Could you check a few things on this model? Use its own coordinates, in mm. Round coordinates to 2 decimals unless told otherwise and drop trailing zeros. Loops run counter-clockwise (first coordinate to the right, second up) from the corner with the lowest first, then second, coordinate; pieces in that order, holes last. Notation, with made-up numbers: M -22,-2.75 L -10,-2.75 A30 cw -10,23.25 Z; hole C 5.25,-18 d4. An arc over 180 degrees is marked long. One line per item, written item: value. Start each with the question number.
Q1. Imagine slicing it at A-A (x = 42). Please give me the cut outline in (y, z).
Q2. I'm going to push flat-ended pins straight in: pin 1 Ø1.6 at (y, z) = (-8.5, 2) entering from +X; pin 2 Ø1.6 at (y, z) = (12.5, 2) entering from -X; pin 3 Ø1.6 at (x, z) = (-1, 1.5) entering from -Y. Where does each tip first touch, or does it pass through?
Q3. Imagine slicing it at B-B (z = 0.7). Give the number of separate pieces and of enclosed holes in the cut face, then the cut area to 3 significant figures.
Q4. Please list where these lines run through material, in increasing order: line 1 along X through (y, z) = (12.25, 0.75); line 2 along X through (y, z) = (0.75, 1.25); line 3 along X through (y, z) = (2.75, 0.8).
from build123d import *

# Parameters (mm, degrees)
SKETCH1_R           = 1.4
BOSS_EXTRUDE1_DEPTH = 3.15
SKETCH2_R           = 1.4
CUT_EXTRUDE1_DEPTH  = 10


with BuildPart() as part:
    # Sketch1 → Boss-Extrude1 (new body)
    with BuildSketch(Plane.XY):
        Polygon((-60.67170061, 10.980201327), (-60.67170061, -7.339798673), (-35.52170061, -7.339798673), (-35.52170061, -7.389798673), (-35.52170061, -10.539798673), (-15.62170061, -10.539798673), (-15.62170061, -7.339798673), (4.47829939, -7.339798673), (4.47829939, -10.539798673), (24.37829939, -10.539798673), (24.37829939, -7.339798673), (44.47829939, -7.339798673), (44.47829939, -10.539798673), (64.37829939, -10.539798673), (64.37829939, -7.339798673), (84.47829939, -7.339798673), (84.47829939, -10.539798673), (104.37829939, -10.539798673), (104.37829939, -7.339798673), (124.47829939, -7.339798673), (124.47829939, -10.539798673), (144.37829939, -10.539798673), (144.37829939, -7.389798673), (144.37829939, -7.339798673), (144.462459505, -7.339798673), (149.52829939, -7.339798673), (149.52829939, 10.980201327), (144.462459505, 10.980201327), (144.37829939, 10.980201327), (144.37829939, 11.030201327), (144.37829939, 14.180201327), (124.47829939, 14.180201327), (124.47829939, 10.980201327), (104.37829939, 10.980201327), (104.37829939, 14.180201327), (84.47829939, 14.180201327), (84.47829939, 10.980201327), (64.37829939, 10.980201327), (64.37829939, 14.180201327), (44.47829939, 14.180201327), (44.47829939, 10.980201327), (24.37829939, 10.980201327), (24.37829939, 14.180201327), (4.47829939, 14.180201327), (4.47829939, 10.980201327), (-15.62170061, 10.980201327), (-15.62170061, 14.180201327), (-35.52170061, 14.180201327), (-35.52170061, 10.980201327), (-35.57170061, 10.980201327), align=None)
        with Locations((-38.12170061, 1.820201327)):
            Circle(SKETCH1_R, mode=Mode.SUBTRACT)
    extrude(amount=BOSS_EXTRUDE1_DEPTH)

    # Sketch2 → Cut-Extrude1 (cut)
    with BuildSketch(Plane.XY.offset(3.15)):
        with Locations((143.385201149, 1.820201327)):
            Circle(SKETCH2_R)
    extrude(amount=-CUT_EXTRUDE1_DEPTH, mode=Mode.SUBTRACT)


solid = part.part
Report:
1. outline: M -7.34,0 L 10.98,0 L 10.98,3.15 L -7.34,3.15 Z
2. pin 1: stops at x = 144.38
2. pin 2: stops at x = -35.52
2. pin 3: stops at y = -7.34
3. separate pieces: 1
3. enclosed holes: 2
3. area: 4,480 mm²
4. line 1: x = -35.52 to -15.62, 4.48 to 24.38, 44.48 to 64.38, 84.48 to 104.38, 124.48 to 144.38
4. line 2: x = -60.67 to -39.02, -37.22 to 142.48, 144.29 to 149.53
4. line 3: x = -60.67 to -39.17, -37.08 to 142.34, 144.43 to 149.53
